from build123d import *

# Parameters (mm, degrees)
SKETCH2_W            = 67.691
SKETCH2_H            = 12.7
SKETCH3_R            = 2.5019
CUT_EXTRUDE1_DEPTH   = 13.7
LPATTERN1_COUNT      = 2
LPATTERN1_PITCH      = 35.921024484
LPATTERN1_COUNT_DIR2 = 2
LPATTERN1_PITCH_DIR2 = 35.921024484
SKETCH5_R            = 15.875
CUT_EXTRUDE2_DEPTH   = 13.7
BOSS_EXTRUDE1_DEPTH  = 15.875
BOSS_EXTRUDE2_DEPTH  = 1.27
CUT_EXTRUDE3_DEPTH   = 13.7
SKETCH13_R           = 4.8387
CUT_EXTRUDE4_DEPTH   = 3.81
SKETCH14_R           = 3.6195
CUT_EXTRUDE5_DEPTH   = 5.715
CUT_EXTRUDE6_DEPTH   = 13.7000001
SKETCH16_R           = 2.413
CUT_EXTRUDE7_DEPTH   = 2.54
CIRPATTERN2_COUNT    = 4


with BuildPart() as part:
    # Sketch2 → Revolve1 (revolve)
    with BuildSketch(Plane(origin=(0, 0, 0), x_dir=(0, 0, -1), z_dir=(1, 0, 0))):
        with Locations((43.3705, 0)):
            Rectangle(SKETCH2_W, SKETCH2_H)
    revolve(axis=Axis((0, 9.434285714, 0), (0, -1, 0)))

    # Sketch3 → Cut-Extrude1 (cut, through all)
    with BuildSketch(Plane(origin=(0, 6.35, 0), x_dir=(1, 0, 0), z_dir=(0, 1, 0))):
        with Locations((17.960512242, 17.960512242)):
            Circle(SKETCH3_R)
    cut_extrude1 = extrude(amount=-CUT_EXTRUDE1_DEPTH, mode=Mode.SUBTRACT)

    # LPattern1: Cut-Extrude1 2 × 2
    with Locations(*[(-j * LPATTERN1_PITCH_DIR2, 0, i * LPATTERN1_PITCH) for i in range(LPATTERN1_COUNT) for j in range(LPATTERN1_COUNT_DIR2) if (i, j) != (0, 0)]):
        add(cut_extrude1, mode=Mode.SUBTRACT)

    # Sketch5 → Cut-Extrude2 (cut, through all)
    with BuildSketch(Plane(origin=(0, 6.35, 0), x_dir=(1, 0, 0), z_dir=(0, 1, 0))):
        with Locations((-35.921024484, -35.921024484)):
            Circle(SKETCH5_R)
    extrude(amount=-CUT_EXTRUDE2_DEPTH, mode=Mode.SUBTRACT)

    # Sketch7 → Boss-Extrude1 (add, symmetric)
    with BuildSketch(Plane(origin=(0, 0, 0), x_dir=(0.707106781, 0, -0.707106781), z_dir=(0.707106781, 0, 0.707106781))):
        Polygon((66.900640303, 6.35), (44.45, 28.800640303), (40.64, 28.800640303), (40.64, 6.35), (44.45, 6.35), (44.45, 23.41248663), (61.51248663, 6.35), align=None)
    extrude(amount=BOSS_EXTRUDE1_DEPTH, both=True)

    # Sketch8 → Boss-Extrude2 (add, symmetric)
    with BuildSketch(Plane(origin=(25.898012242, 36.625320151, -25.898012242), x_dir=(0.866025404, -0.40824829, 0.288675135), z_dir=(0.5, 0.707106781, -0.5))):
        Polygon((37.681578612, 25.793492955), (11.757812168, 44.124364002), (-6.573058879, 18.200597557), (-5.743498353, 17.614009684), (-5.156910479, 18.44357021), (12.000784821, 42.708215602), (36.265430213, 25.550520302), (19.107734913, 1.28587491), (18.521147039, 0.456314384), (19.350707566, -0.130273489), align=None)
    extrude(amount=BOSS_EXTRUDE2_DEPTH, both=True)

    # Sketch12 → Cut-Extrude3 (cut, through all)
    with BuildSketch(Plane(origin=(0, 6.35, 0), x_dir=(1, 0, 0), z_dir=(0, 1, 0))):
        Polygon((73.406, -11.43), (58.801, -11.43), (58.801, -9.652), (71.628, -9.652), (71.628, 9.652), (58.801, 9.652), (58.801, 11.43), (73.406, 11.43), align=None)
    cut_extrude3 = extrude(amount=-CUT_EXTRUDE3_DEPTH, mode=Mode.SUBTRACT)

    # Sketch13 → Cut-Extrude4 (cut)
    with BuildSketch(Plane(origin=(77.216, 0, 0), x_dir=(0, 0, -1), z_dir=(1, 0, 0))):
        Circle(SKETCH13_R)
    cut_extrude4 = extrude(amount=-CUT_EXTRUDE4_DEPTH, mode=Mode.SUBTRACT)

    # Sketch14 → Cut-Extrude5 (cut)
    with BuildSketch(Plane(origin=(71.628, 0, 0), x_dir=(0, 0, -1), z_dir=(1, 0, 0))):
        Circle(SKETCH14_R)
    cut_extrude5 = extrude(amount=-CUT_EXTRUDE5_DEPTH, mode=Mode.SUBTRACT)

    # Sketch15 → Cut-Extrude6 (cut, through all)
    with BuildSketch(Plane(origin=(0, 6.35, 0), x_dir=(1, 0, 0), z_dir=(0, 1, 0))):
        with BuildLine():
            Line((73.406, 11.43), (76.365343946, 11.43))
            ThreePointArc((76.365343946, 11.43), (77.216, 0), (76.365343946, -11.43))
            Line((76.365343946, -11.43), (73.406, -11.43))
            Line((73.406, -11.43), (73.406, 11.43))
        make_face()
    cut_extrude6 = extrude(amount=-CUT_EXTRUDE6_DEPTH, mode=Mode.SUBTRACT)

    # Sketch16 → Cut-Extrude7 (cut)
    with BuildSketch(Plane(origin=(65.913, 0, 0), x_dir=(0, 0, -1), z_dir=(1, 0, 0))):
        Circle(SKETCH16_R)
    cut_extrude7 = extrude(amount=-CUT_EXTRUDE7_DEPTH, mode=Mode.SUBTRACT)

    # CirPattern2: Cut-Extrude3, Cut-Extrude4, Cut-Extrude5, Cut-Extrude6, Cut-Extrude7 ×4 about axis
    cirpattern2_axis = Axis((0, 0, 0), (0, 1, 0))
    for i in range(1, CIRPATTERN2_COUNT):
        add(cut_extrude3.rotate(cirpattern2_axis, i * 360 / CIRPATTERN2_COUNT), mode=Mode.SUBTRACT)
        add(cut_extrude4.rotate(cirpattern2_axis, i * 360 / CIRPATTERN2_COUNT), mode=Mode.SUBTRACT)
        add(cut_extrude5.rotate(cirpattern2_axis, i * 360 / CIRPATTERN2_COUNT), mode=Mode.SUBTRACT)
        add(cut_extrude6.rotate(cirpattern2_axis, i * 360 / CIRPATTERN2_COUNT), mode=Mode.SUBTRACT)
        add(cut_extrude7.rotate(cirpattern2_axis, i * 360 / CIRPATTERN2_COUNT), mode=Mode.SUBTRACT)


solid = part.part
Work out the finished part from the listing and answer in its coordinate system (mm). A direction names the side the tool comes from. Give positions to 0.01 mm unless a question says otherwise; leave off trailing zeros. Order: outer loops, then holes, each group sorted by start corner. A loop starts at its lowest first (then second) coordinate and runs counter-clockwise, first axis right, second up. Notation, with made-up numbers: (-31, 82.25) -> (20, 82.25) arc R19 ccw to (20, 119.25) -> close; hole circle Ø2 at (9, 62.25). An arc over 180 degrees is marked (long way). Answer as a JSON object with one key per item and string values. Group by question number.
1. Section C-C on y = 10 is taken. Determine the outline of the cut face in (x, z).
2. Section D-D on z = 38.5 is taken. Determine the outline of the cut face in (x, y), plus the area to 3 significant figures.
3. A tool of negligible diameter and unlimited length cuts with its end or side. For faces 5 (the flat face through (31.59, 14.76, -31.27)), 6 (the cylindrical face through (0.47, 3.59, -68.81)), 7 (the cylindrical face through (-0.47, 3.59, 68.81)), 8 (the cylindrical face through (64.661, -1.468, 1.915)), from which of +Z, -Z, +X, -X, +Y, -Y can it reach the whole face along a straight path? Write none if from no direction.
4. The mould has two halves that part along X. Classify faces 1 (the cylindrical face through (54.111, 0.089, -55.085)), 2 (the cylindrical face through (68.81, 3.59, 0.47)), 3 (the cylindrical face through (19.306, 0.089, 15.851)), 4 (the flat face through (-9.652, 0, 65)): released by +X, released by -X, zero draft, split by the parting line, or undercut.
5. Flat-ended cylindrical pins translate along their axes: pin 1 Ø6.5 at (x, y) = (-3, -1.5) entering from -Z; pin 2 Ø7.5 at (y, z) = (0, 0) entering from +X; pin 3 Ø10 at (x, y) = (-68.5, 1) entering from -Z. Find the tip coordinate at first contact, or state that the pin passes through.
6. Consider line 1 along Y through (x, z) = (65.4, 0); line 2 along Y through (x, z) = (0, -68.9); line 3 along Y through (x, z) = (3.5, -10.5). Determine where each line is inside the solid, lowest interval first. Write a range as [from, to].
Result sheet:
{
 "1": {"outline": "(17.51, -39.96) -> (20.21, -42.66) -> (42.66, -20.21) -> (39.96, -17.51) -> close; (29.69, -52.14) -> (34.77, -57.22) -> (35.49, -56.5) -> (34.22, -55.23) -> (55.23, -34.22) -> (56.5, -35.49) -> (57.22, -34.77) -> (52.14, -29.69) -> close"},
 "2": {"outline": "(-66.93, -6.35) -> (-51.59, -6.35) -> (-51.59, 6.35) -> (-66.93, 6.35) -> close; (-20.26, -6.35) -> (66.93, -6.35) -> (66.93, 6.35) -> (-20.26, 6.35) -> close", "area": "1,300 mm^2"},
 "3": {"face 5": "none", "face 6": "-Z", "face 7": "+Z", "face 8": "+X"},
 "4": {"face 1": "released by +X", "face 2": "zero draft", "face 3": "undercut", "face 4": "undercut"},
 "5": {"pin 1": "stops at z = -71.63", "pin 2": "stops at x = 71.63", "pin 3": "stops at z = -43.93"},
 "6": {"line 1": "y = [-6.35, -2.41], [2.41, 6.35]", "line 2": "y = [-6.35, -3.62], [3.62, 6.35]", "line 3": "y = [-6.35, 6.35]"}
}
